```python
from build123d import *

# Parameters (mm, degrees)
SKETCH1_W           = 650
SKETCH1_H           = 125
BOSS_EXTRUDE1_DEPTH = 10
SKETCH2_R           = 10
CUT_EXTRUDE2_DEPTH  = 10
SKETCH3_R           = 10
CUT_EXTRUDE3_DEPTH  = 10
SKETCH8_R           = 3
CUT_EXTRUDE5_DEPTH  = 20
CUT_EXTRUDE7_DEPTH  = 30
CUT_EXTRUDE8_DEPTH  = 30
BOSS_EXTRUDE5_DEPTH = 20
SKETCH12_W          = 10
SKETCH12_H          = 10
CUT_EXTRUDE9_DEPTH  = 5
SKETCH13_R          = 3
CUT_EXTRUDE10_DEPTH = 5
FILLET3_R           = 50
FILLET5_R           = 40
FILLET6_R           = 50
FILLET7_R           = 40
SKETCH14_W          = 133
SKETCH14_H          = 20
CUT_EXTRUDE11_DEPTH = 80


with BuildPart() as part:
    # Sketch1 → Boss-Extrude1 (new body)
    with BuildSketch(Plane.XY):
        with Locations((277.89592831, 25.809681948)):
            Rectangle(SKETCH1_W, SKETCH1_H)
    extrude(amount=BOSS_EXTRUDE1_DEPTH)

    # Sketch2 → Cut-Extrude2 (cut)
    with BuildSketch(Plane.XY.offset(10)):
        with Locations((-7.10407169, 48.309681948)):
            Circle(SKETCH2_R)
    extrude(amount=-CUT_EXTRUDE2_DEPTH, mode=Mode.SUBTRACT)

    # Sketch3 → Cut-Extrude3 (cut)
    with BuildSketch(Plane.XY.offset(10)):
        with Locations((562.89592831, 48.309681948)):
            Circle(SKETCH3_R)
    extrude(amount=-CUT_EXTRUDE3_DEPTH, mode=Mode.SUBTRACT)

    # Sketch8 → Cut-Extrude5 (cut)
    with BuildSketch(Plane.XY.offset(10)):
        with Locations((177.509070801, 48.309681948)):
            Circle(SKETCH8_R)
        with Locations((377.89592831, 48.309681948)):
            Circle(SKETCH8_R)
    extrude(amount=-CUT_EXTRUDE5_DEPTH, mode=Mode.SUBTRACT)

    # Sketch10 → Cut-Extrude7 (cut)
    with BuildSketch(Plane(origin=(0, 88.309681948, 0), x_dir=(1, 0, 0), z_dir=(0, 1, 0))):
        Polygon((277.89592831, -3), (307.89592831, -3), (307.89592831, -7), (277.89592831, -7), (247.89592831, -7), (247.89592831, -3), align=None)
    extrude(amount=-CUT_EXTRUDE7_DEPTH, mode=Mode.SUBTRACT)

    # Sketch9 → Cut-Extrude8 (cut)
    with BuildSketch(Plane.XY.offset(10)):
        Polygon((277.89592831, 68.309681948), (257.89592831, 68.309681948), (257.89592831, 88.309681948), (297.89592831, 88.309681948), (297.89592831, 68.309681948), align=None)
    extrude(amount=-CUT_EXTRUDE8_DEPTH, mode=Mode.SUBTRACT)

    # Sketch7 → Boss-Extrude5 (add)
    with BuildSketch(Plane.XY.offset(10)):
        Polygon((160.89592831, 25.309681948), (158.89592831, 25.309681948), (158.89592831, -34.690318052), (98.89592831, -34.690318052), (98.89592831, 25.309681948), (96.89592831, 25.309681948), (96.89592831, -36.690318052), (160.89592831, -36.690318052), align=None)
        Polygon((89.89592831, 25.309681948), (91.89592831, 25.309681948), (91.89592831, -36.690318052), (27.89592831, -36.690318052), (27.89592831, 25.309681948), (29.89592831, 25.309681948), (29.89592831, -34.690318052), (89.89592831, -34.690318052), align=None)
    extrude(amount=BOSS_EXTRUDE5_DEPTH)

    # Sketch12 → Cut-Extrude9 (cut)
    with BuildSketch(Plane(origin=(602.89592831, 0, 0), x_dir=(0, 0, -1), z_dir=(1, 0, 0))):
        with Locations((-5, 30.809681948)):
            Rectangle(SKETCH12_W, SKETCH12_H)
    extrude(amount=-CUT_EXTRUDE9_DEPTH, mode=Mode.SUBTRACT)

    # Sketch13 → Cut-Extrude10 (cut)
    with BuildSketch(Plane(origin=(597.89592831, 0, 0), x_dir=(0, 0, -1), z_dir=(1, 0, 0))):
        with Locations((-5, 30.809681948)):
            Circle(SKETCH13_R)
    extrude(amount=-CUT_EXTRUDE10_DEPTH, mode=Mode.SUBTRACT)

    # Fillet3
    fillet3_edges = [part.edges().sort_by_distance(p)[0] for p in [
        (602.89592831, -36.690318052, 5),
    ]]
    fillet(fillet3_edges, radius=FILLET3_R)

    # Fillet5
    fillet5_edges = [part.edges().sort_by_distance(p)[0] for p in [
        (602.89592831, 88.309681948, 5),
    ]]
    fillet(fillet5_edges, radius=FILLET5_R)

    # Fillet6
    fillet6_edges = [part.edges().sort_by_distance(p)[0] for p in [
        (-47.10407169, -36.690318052, 5),
    ]]
    fillet(fillet6_edges, radius=FILLET6_R)

    # Fillet7
    fillet7_edges = [part.edges().sort_by_distance(p)[0] for p in [
        (-47.10407169, 88.309681948, 5),
    ]]
    fillet(fillet7_edges, radius=FILLET7_R)

    # Sketch14 → Cut-Extrude11 (cut)
    with BuildSketch(Plane.XZ.offset(36.690318052)):
        with Locations((94.39592831, 20)):
            Rectangle(SKETCH14_W, SKETCH14_H)
    extrude(amount=-CUT_EXTRUDE11_DEPTH, mode=Mode.SUBTRACT)


solid = part.part
```
For this review, take the finished solid that the model builds, in its own axes (mm). A direction names the side the tool comes from. Round coordinates to 2 decimals unless told otherwise and drop trailing zeros. Write each loop counter-clockwise with the first axis right and the second up, starting at its lowest first coordinate (ties: lowest second). Pieces come first, ordered by that corner, then holes. Notation, with made-up numbers: M 30.25,44.5 L 84.25,44.5 A17 cw 84.25,68.5 Z; hole C 9.25,49 d9. An arc over 180 degrees is marked long. One line per item, written item: value. Start each with the question number.
(1) We need section B-B (y = -17). Give the boundary of the cut face in (x, z), and give its area (3 significant figures).
(2) Machinability: for faces 4 (the flat face through (277, 67, 7)), 5 (the flat face through (429, 88.31, 5)), 6 (the flat face through (597.896, 33.1, 2.8)), which of the approach directions +Z, -Z, +X, -X, +Y, -Y give a long, thin tool a straight path to every point of the face, cutting with its end or side? Answer none if there is none.
(3) We need section A-A (z = 5). Give the boundary of the cut face in (x, y), and give its area (3 significant figures).
(4) Wall thickness on line 1 (X direction, y = 42, z = 4); line 2 (X direction, y = 28.5, z = 2.5); line 3 (X direction, y = 66.5, z = 6.5): over which ranges is each line inside the solid? List them lowest first.
(5) Insertion check: pin 1 (24 mm diameter, centred on x = 266, y = 78.5, fed in from +Z); pin 2 (2.5 mm diameter, centred on y = 74, z = 1.5, fed in from +X); pin 3 (5.5 mm diameter, centred on x = 177.51, y = 48.31, fed in from -Z); pin 4 (1.5 mm diameter, centred on y = 76, z = 8.5, fed in from +X). Each pin has a flat end and moves straight along its axis. Give the tip position at first contact, or say it passes through.
(6) The part is to be moulded in two halves that separate along Z. For faces 1 (the flat face through (273, 27, 10)), 2 (the flat face through (278, 67, 3)), 3 (the flat face through (-47.104, 31, 5)), say which applies: released by +Z, released by -Z, zero draft, split by the parting line, or undercut.
Result:
1. outline: M -36.87,0 L 592.66,0 L 592.66,10 L -36.87,10 Z
1. area: 6,300 mm²
2. face 4: +Y
2. face 5: +Z, -Z, +X, -X, +Y
2. face 6: +Z, -Z, +X
3. outline: M -47.1,13.31 A50 ccw 2.9,-36.69 L 552.9,-36.69 A50 ccw 602.9,13.31 L 602.9,25.81 L 597.9,25.81 L 597.9,27.81 L 592.9,27.81 L 592.9,33.81 L 597.9,33.81 L 597.9,35.81 L 602.9,35.81 L 602.9,48.31 A40 ccw 562.9,88.31 L 307.9,88.31 L 307.9,58.31 L 247.9,58.31 L 247.9,88.31 L -7.1,88.31 A40 ccw -47.1,48.31 Z; hole C -7.1,48.31 d20; hole C 177.51,48.31 d6; hole C 377.9,48.31 d6; hole C 562.9,48.31 d20
3. area: 76,900 mm²
4. line 1: -47.1 to -14.86, 0.65 to 555.14, 570.65 to 602.9
4. line 2: -47.1 to 597.9
4. line 3: -42.73 to 247.9, 307.9 to 598.52
5. pin 1: z = 10
5. pin 2: x = 594.56
5. pin 3: through
5. pin 4: x = 592.46
6. face 1: released by +Z
6. face 2: undercut
6. face 3: zero draft
